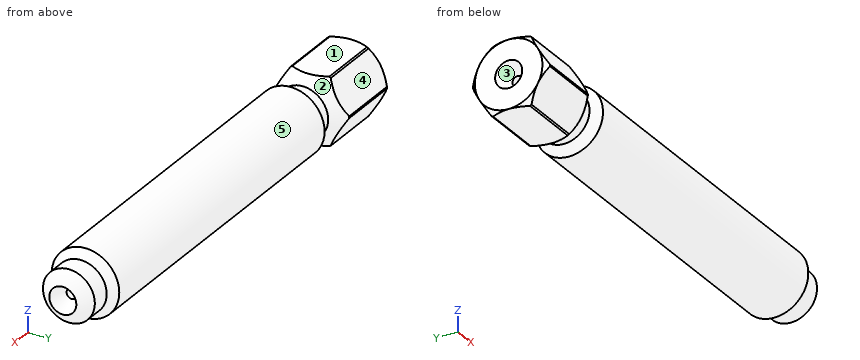
```python
from build123d import *

# Parameters (mm, degrees)
SKETCH2_OUTSIDE_W  = 23.076
SKETCH2_OUTSIDE_H  = 23.077
CUT_EXTRUDE1_DEPTH = 57.16575
SKETCH3_OUTSIDE_W  = 21.43
SKETCH3_OUTSIDE_H  = 22.658
SKETCH3_OUTSIDE_R  = 4.5212
CUT_EXTRUDE2_DEPTH = 57.16575


with BuildPart() as part:
    # Sketch1 → Revolve1 (revolve)
    with BuildSketch(Plane.XY):
        with BuildLine():
            Line((-4.73075, 3.96875), (-44.45, 3.96875))
            Line((-44.45, 3.96875), (-45.43425, 2.9845))
            Line((-45.43425, 2.9845), (-46.76775, 2.9845))
            Line((-46.76775, 2.9845), (-48.54575, 4.7625))
            Line((-48.54575, 4.7625), (-55.372, 4.7625))
            Line((-55.372, 4.7625), (-56.16575, 3.96875))
            Line((-56.16575, 3.96875), (-56.16575, 0))
            Line((-56.16575, 0), (0, 0))
            ThreePointArc((0, 0), (-0.402232402, 1.703883799), (-1.524, 3.048))
            Line((-1.524, 3.048), (-3.81, 3.048))
            Line((-3.81, 3.048), (-4.73075, 3.96875))
        make_face()
    revolve(axis=Axis((1.163601772, 0, 0), (-1, 0, 0)))

    # Sketch2 outside → Cut-Extrude1 (cut, through all)
    with BuildSketch(Plane.ZY.offset(56.16575)):
        with Locations((0, -0.0005)):
            Rectangle(SKETCH2_OUTSIDE_W, SKETCH2_OUTSIDE_H)
        Polygon((0, -4.582717762), (3.96875, -2.291358881), (3.96875, 2.291358881), (0, 4.582717762), (-3.96875, 2.291358881), (-3.96875, -2.291358881), align=None, mode=Mode.SUBTRACT)
    extrude(amount=-CUT_EXTRUDE1_DEPTH, mode=Mode.SUBTRACT)

    # Sketch3 outside → Cut-Extrude2 (cut, through all)
    with BuildSketch(Plane.ZY.offset(56.16575)):
        Rectangle(SKETCH3_OUTSIDE_W, SKETCH3_OUTSIDE_H)
        Circle(SKETCH3_OUTSIDE_R, mode=Mode.SUBTRACT)
    extrude(amount=-CUT_EXTRUDE2_DEPTH, mode=Mode.SUBTRACT)

    # Sketch4 → Cut-Revolve1 (revolve, cut)
    with BuildSketch(Plane.XY):
        with BuildLine():
            Line((-0.346483904, 1.5875), (-2.065003064, 0.5953125))
            Line((-2.065003064, 0.5953125), (-3.255628064, 0.5953125))
            Line((-3.255628064, 0.5953125), (-3.599331896, 0))
            Line((-3.599331896, 0), (0, 0))
            ThreePointArc((0, 0), (-0.087628691, 0.812435743), (-0.346483904, 1.5875))
        make_face()
        Polygon((-56.16575, 0), (-52.912902007, 0), (-53.256605839, 0.5953125), (-54.447230839, 0.5953125), (-56.16575, 1.5875), align=None)
    revolve(axis=Axis((1.163601772, 0, 0), (-1, 0, 0)), mode=Mode.SUBTRACT)


solid = part.part
```
Input: part model. Units: mm. Frame: model coordinates. Face numbers are marked on the shaded views. A direction names the side the tool comes from. Round coordinates to 2 decimals unless told otherwise and drop trailing zeros. Loops run counter-clockwise (first coordinate to the right, second up) from the corner with the lowest first, then second, coordinate; pieces in that order, holes last. Notation, with made-up numbers: (-2, -7.75) -> (13, -7.75) arc R20 ccw to (13, 18.25) -> close; hole circle Ø11 at (2, 7). An arc over 180 degrees is marked (long way). Use one line per item in the form item = value. Start each with the question number.
Item 1: Set-up query: the marked faces 1 and 2. Return all of +Z, -Z, +X, -X, +Y, -Y with unobstructed straight access to the full face (end or side cutting, diameter ignored); none if empty.
Item 2: Mould query, pull axis Z, two halves, no side actions, for the marked faces 3, 4 and 5. Classes: pulls with the +Z half, pulls with the -Z half, needs draft (parallel to the pull), parting line crosses it, or undercut.
Item 3: Section query A-A on x = -33.5. Return the cut outline in (y, z).
Item 4: Contact query for flat-ended pins moving along their axis: pin 1 Ø2 at (x, y) = (-28, 2.5) entering from +Z; pin 2 Ø2 at (y, z) = (-2.5, 1.5) entering from +X; pin 3 Ø1 at (y, z) = (0, 0) entering from -X. Output: stop coordinate, or through.
Item 5: Material intervals for L1, parallel to Z at x = -53.75, y = 0; L2, parallel to Y at x = -53.7, z = 0; L3, parallel to Z at x = -2.95, y = 0, sorted ascending. Write a range as from..to.
Ans:
q1.face_1 = +Z, +X, -X, +Y, -Y
q1.face_2 = none
q2.face_3 = undercut
q2.face_4 = pulls with the +Z half
q2.face_5 = parting line crosses it
q3.outline = circle Ø7.94 at (0, 0)
q4.pin_1 = 3.67
q4.pin_2 = -0.52
q4.pin_3 = -53.2
q5.L1 = -3.97..-0.6, 0.6..3.97
q5.L2 = -4.52..-0.6, 0.6..4.52
q5.L3 = -3.05..-0.6, 0.6..3.05
